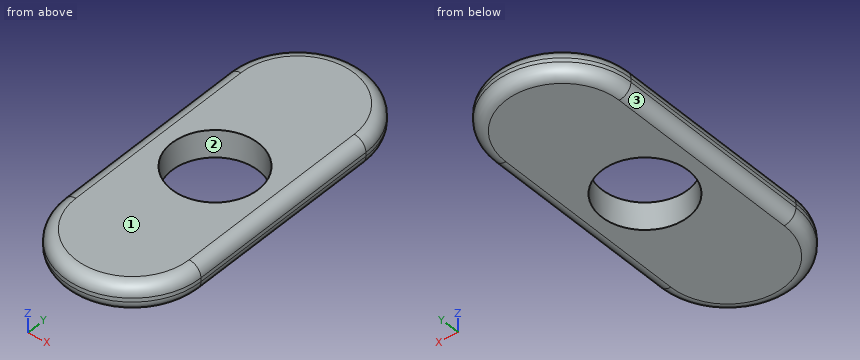
```python
from build123d import *

# Parameters (mm, degrees)
F1_DEPTH = 7
F2_D     = 22.1
F3_R     = 3


with BuildPart() as f1:
    # F0 (on Top) → F1 (new body)
    with BuildSketch(Plane.XY):
        Polygon((-0.2911061255, 6.1655282974), (-17.7911061255, 31.1655282974), (-17.7911061255, -18.8344717026), align=None)
        with BuildLine():
            ThreePointArc((17.2088938745, 31.1655282974), (-0.2911061255, 48.6655282974), (-17.7911061255, 31.1655282974))
            Line((-17.7911061255, 31.1655282974), (17.2088938745, 31.1655282974))
        make_face()
        Polygon((17.2088938745, 31.1655282974), (-17.7911061255, 31.1655282974), (-0.2911061255, 6.1655282974), align=None)
        Polygon((-0.2911061255, 6.1655282974), (-17.7911061255, -18.8344717026), (17.2088938745, -18.8344717026), align=None)
        with BuildLine():
            Line((17.2088938745, -18.8344717026), (-17.7911061255, -18.8344717026))
            ThreePointArc((-17.7911061255, -18.8344717026), (-0.2911061255, -36.3344717026), (17.2088938745, -18.8344717026))
        make_face()
        Polygon((17.2088938745, -18.8344717026), (17.2088938745, 31.1655282974), (-0.2911061255, 6.1655282974), align=None)
    extrude(amount=F1_DEPTH)

    # F2 (through all)
    with Locations(Plane(origin=(0, 0, 0), x_dir=(1, 0, 0), z_dir=(0, 0, -1))):
        with Locations((-0.2911061255, -6.1655282974)):
            Hole(F2_D / 2)

    # F3
    f3_edges = [f1.edges().sort_by_distance(p)[0] for p in [
        (17.208894, -18.834472, 3.5),
        (17.208894, 31.165528, 3.5),
        (17.208894, 6.165528, 0),
        (17.208894, 6.165528, 7),
        (-17.791106, -18.834472, 3.5),
        (-0.291106, -36.334472, 0),
        (-0.291106, -36.334472, 7),
        (-17.791106, 31.165528, 3.5),
        (-17.791106, 6.165528, 0),
        (-17.791106, 6.165528, 7),
    ]]
    fillet(f3_edges, radius=F3_R)


solid = f1.part
```
Check sheet for the modelled part. Datum: model origin and axes. Units: mm. Face numbers are marked on the shaded views. Round coordinates to 2 decimals unless told otherwise and drop trailing zeros. Order: outer loops, then holes, each group sorted by start corner. A loop starts at its lowest first (then second) coordinate and runs counter-clockwise, first axis right, second up. Notation, with made-up numbers: M -29,50.25 L -20,50.25 A21 cw -20,77.25 Z; hole C 49,86 d8. An arc over 180 degrees is marked long. Answer in a Markdown table with one row per item.
(1) Material ranges on line 1 along Y through (x, z) = (-4, 1); line 2 along X through (y, z) = (10, 2.75); line 3 along Y through (x, z) = (-1, 4), recorded low to high. Write a range as from..to.
Findings:
| item | result |
|---|---|
| line 1 | y = -35.15..-4.24, 16.57..47.49 |
| line 2 | x = -17.78..-10.65, 10.07..17.2 |
| line 3 | y = -36.32..-4.86, 17.19..48.65 |
(2) Draft check along X on the marked faces 1, 2 and 3. Enter one of: +X half, -X half, draft (parallel to the pull), parting line (faces both ways), or undercut.
Findings:
| item | result |
|---|---|
| face 1 | draft |
| face 2 | undercut |
| face 3 | -X half |
(3) Gauge pin test, flat ends, axial feed: pin 1 (4 mm diameter, centred on y = 4.5, z = 2, fed in from -X); pin 2 (2 mm diameter, centred on x = 3, z = 0.5, fed in from -Y); pin 3 (2 mm diameter, centred on x = 11.5, z = 3, fed in from -Y). Record the tip position at first contact, or that the pin passes through.
Findings:
| item | result |
|---|---|
| pin 1 | stops at x = -17.79 |
| pin 2 | stops at y = -35.64 |
| pin 3 | stops at y = -32.61 |
(4) Section check D-D on z = 1.5. Record the boundary of the cut face in (x, y), plus the area to 3 significant figures.
Findings:
| item | result |
|---|---|
| outline | M -17.39,-18.83 A17.1 ccw 16.81,-18.83 L 16.81,31.17 A17.1 ccw -17.39,31.17 Z; hole C -0.29,6.17 d22.1 |
| area | 2,240 mm^2 |
(5) Section check A-A on y = 9. Record the boundary of the cut face in (x, z).
Findings:
| item | result |
|---|---|
| outline | M -17.79,3 A3 ccw -14.79,0 L -10.97,0 L -10.97,7 L -14.79,7 A3 ccw -17.79,4 Z; M 10.39,0 L 14.21,0 A3 ccw 17.21,3 L 17.21,4 A3 ccw 14.21,7 L 10.39,7 Z |
(6) Section check C-C on y = 23. Record the boundary of the cut face in (x, z).
Findings:
| item | result |
|---|---|
| outline | M -17.79,3 A3 ccw -14.79,0 L 14.21,0 A3 ccw 17.21,3 L 17.21,4 A3 ccw 14.21,7 L -14.79,7 A3 ccw -17.79,4 Z |
(7) Section check B-B on z = 5.25. Record the boundary of the cut face in (x, y).
Findings:
| item | result |
|---|---|
| outline | M -17.52,-18.83 A17.23 ccw 16.94,-18.83 L 16.94,31.17 A17.23 ccw -17.52,31.17 Z; hole C -0.29,6.17 d22.1 |
